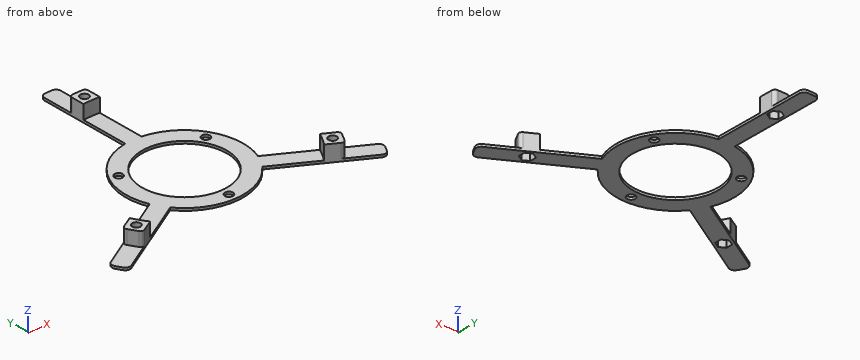
```python
from build123d import *

# Parameters (mm, degrees)
F0_R     = 2.5
F1_DEPTH = 1.5
F2_DEPTH = 10
F3_R     = 2
F4_R     = 3
F5_DEPTH = 4.5


with BuildPart() as f1:
    # F0 (on Top) → F1 (new body)
    with BuildSketch(Plane.XY):
        with BuildLine():
            Line((84.6583836258, -43.1040378836), (67.3074069841, -33.0864468488))
            ThreePointArc((67.3074069841, -33.0864468488), (64.9519052838, -37.5), (62.3074069841, -41.7467008867))
            Line((62.3074069841, -41.7467008867), (79.6583836258, -51.7642919214))
            ThreePointArc((79.6583836258, -51.7642919214), (82.2724133595, -47.5), (84.6583836258, -43.1040378836))
        make_face()
        with BuildLine():
            ThreePointArc((62.3074069841, -41.7467008867), (64.9519052838, -37.5), (67.3074069841, -33.0864468488))
            Line((67.3074069841, -33.0864468488), (62.3074069841, -41.7467008867))
        make_face()
        with BuildLine():
            Line((67.3074069841, -33.0864468488), (58.6248608016, -28.0735764731))
            ThreePointArc((58.6248608016, -28.0735764731), (56.291651246, -32.5), (53.6248608016, -36.733830511))
            Line((53.6248608016, -36.733830511), (62.3074069841, -41.7467008867))
            Line((62.3074069841, -41.7467008867), (67.3074069841, -33.0864468488))
        make_face()
        Polygon((63.9661338928, -36.9308646221), (60.4661338928, -38.9515905642), (56.9661338928, -36.9308646221), (56.9661338928, -32.8894127377), (60.4661338928, -30.8686867956), (63.9661338928, -32.8894127377), align=None, mode=Mode.SUBTRACT)
        with BuildLine():
            Line((58.6248608016, -28.0735764731), (33.3747469625, -13.4954164511))
            ThreePointArc((33.3747469625, -13.4954164511), (31.1769145362, -18), (28.3747469625, -22.1556704889))
            Line((28.3747469625, -22.1556704889), (53.6248608016, -36.733830511))
            ThreePointArc((53.6248608016, -36.733830511), (56.291651246, -32.5), (58.6248608016, -28.0735764731))
        make_face()
        with BuildLine():
            Line((33.3747469625, -13.4954164511), (24.596379794, -8.4272238033))
            ThreePointArc((24.596379794, -8.4272238033), (22.5166604984, -13), (19.596379794, -17.0874778411))
            Line((19.596379794, -17.0874778411), (28.3747469625, -22.1556704889))
            ThreePointArc((28.3747469625, -22.1556704889), (31.1769145362, -18), (33.3747469625, -13.4954164511))
        make_face()
        with BuildLine():
            ThreePointArc((5, 25.5147016443), (20.0748598999, 16.5227116419), (26, 0))
            ThreePointArc((26, 0), (25.6466944716, -4.2716580713), (24.596379794, -8.4272238033))
            Line((24.596379794, -8.4272238033), (33.3747469625, -13.4954164511))
            ThreePointArc((33.3747469625, -13.4954164511), (35.3375925231, -6.8741948383), (36, 0))
            ThreePointArc((36, 0), (27.1661554144, 23.622023622), (5, 35.65108694))
            Line((5, 35.65108694), (5, 25.5147016443))
        make_face()
        with Locations((26.8467875173, 15.5)):
            Circle(F0_R, mode=Mode.SUBTRACT)
        with BuildLine():
            Line((28.3747469625, -22.1556704889), (19.596379794, -17.0874778411))
            ThreePointArc((19.596379794, -17.0874778411), (0, -26), (-19.596379794, -17.0874778411))
            Line((-19.596379794, -17.0874778411), (-28.3747469625, -22.1556704889))
            ThreePointArc((-28.3747469625, -22.1556704889), (0, -36), (28.3747469625, -22.1556704889))
        make_face()
        with Locations((0, -31)):
            Circle(F0_R, mode=Mode.SUBTRACT)
        with BuildLine():
            ThreePointArc((-28.3747469625, -22.1556704889), (-31.1769145362, -18), (-33.3747469625, -13.4954164511))
            Line((-33.3747469625, -13.4954164511), (-58.6248608016, -28.0735764731))
            ThreePointArc((-58.6248608016, -28.0735764731), (-56.291651246, -32.5), (-53.6248608016, -36.733830511))
            Line((-53.6248608016, -36.733830511), (-28.3747469625, -22.1556704889))
        make_face()
        with BuildLine():
            ThreePointArc((-19.596379794, -17.0874778411), (-22.5166604984, -13), (-24.596379794, -8.4272238033))
            Line((-24.596379794, -8.4272238033), (-33.3747469625, -13.4954164511))
            ThreePointArc((-33.3747469625, -13.4954164511), (-31.1769145362, -18), (-28.3747469625, -22.1556704889))
            Line((-28.3747469625, -22.1556704889), (-19.596379794, -17.0874778411))
        make_face()
        with BuildLine():
            ThreePointArc((-53.6248608016, -36.733830511), (-56.291651246, -32.5), (-58.6248608016, -28.0735764731))
            Line((-58.6248608016, -28.0735764731), (-67.3074069841, -33.0864468488))
            Line((-67.3074069841, -33.0864468488), (-62.3074069841, -41.7467008867))
            Line((-62.3074069841, -41.7467008867), (-53.6248608016, -36.733830511))
        make_face()
        Polygon((-63.9661338928, -32.8894127377), (-60.4661338928, -30.8686867956), (-56.9661338928, -32.8894127377), (-56.9661338928, -36.9308646221), (-60.4661338928, -38.9515905642), (-63.9661338928, -36.9308646221), align=None, mode=Mode.SUBTRACT)
        with BuildLine():
            Line((-62.3074069841, -41.7467008867), (-67.3074069841, -33.0864468488))
            ThreePointArc((-67.3074069841, -33.0864468488), (-64.9519052838, -37.5), (-62.3074069841, -41.7467008867))
        make_face()
        with BuildLine():
            ThreePointArc((-62.3074069841, -41.7467008867), (-64.9519052838, -37.5), (-67.3074069841, -33.0864468488))
            Line((-67.3074069841, -33.0864468488), (-84.6583836258, -43.1040378836))
            ThreePointArc((-84.6583836258, -43.1040378836), (-82.2724133595, -47.5), (-79.6583836258, -51.7642919214))
            Line((-79.6583836258, -51.7642919214), (-62.3074069841, -41.7467008867))
        make_face()
        with BuildLine():
            ThreePointArc((-24.596379794, -8.4272238033), (-22.5166604984, 13), (-5, 25.5147016443))
            Line((-5, 25.5147016443), (-5, 35.65108694))
            ThreePointArc((-5, 35.65108694), (-31.1769145362, 18), (-33.3747469625, -13.4954164511))
            Line((-33.3747469625, -13.4954164511), (-24.596379794, -8.4272238033))
        make_face()
        with Locations((-26.8467875173, 15.5)):
            Circle(F0_R, mode=Mode.SUBTRACT)
        with BuildLine():
            ThreePointArc((-5, 25.5147016443), (0, 26), (5, 25.5147016443))
            Line((5, 25.5147016443), (5, 35.65108694))
            ThreePointArc((5, 35.65108694), (0, 36), (-5, 35.65108694))
            Line((-5, 35.65108694), (-5, 25.5147016443))
        make_face()
        with BuildLine():
            ThreePointArc((-5, 35.65108694), (0, 36), (5, 35.65108694))
            Line((5, 35.65108694), (5, 64.8074069841))
            ThreePointArc((5, 64.8074069841), (0, 65), (-5, 64.8074069841))
            Line((-5, 64.8074069841), (-5, 35.65108694))
        make_face()
        with BuildLine():
            ThreePointArc((-5, 64.8074069841), (0, 65), (5, 64.8074069841))
            Line((5, 64.8074069841), (5, 74.8331477355))
            Line((5, 74.8331477355), (-5, 74.8331477355))
            Line((-5, 74.8331477355), (-5, 64.8074069841))
        make_face()
        Polygon((0, 73.8617292441), (3.5, 71.8410033019), (3.5, 67.7995514176), (0, 65.7788254755), (-3.5, 67.7995514176), (-3.5, 71.8410033019), align=None, mode=Mode.SUBTRACT)
        with BuildLine():
            Line((-5, 74.8331477355), (5, 74.8331477355))
            ThreePointArc((5, 74.8331477355), (0, 75), (-5, 74.8331477355))
        make_face()
        with BuildLine():
            ThreePointArc((-5, 74.8331477355), (0, 75), (5, 74.8331477355))
            Line((5, 74.8331477355), (5, 94.8683298051))
            ThreePointArc((5, 94.8683298051), (0, 95), (-5, 94.8683298051))
            Line((-5, 94.8683298051), (-5, 74.8331477355))
        make_face()
        Polygon((56.9661338928, -36.9308646221), (60.4661338928, -38.9515905642), (63.9661338928, -36.9308646221), (63.9661338928, -32.8894127377), (60.4661338928, -30.8686867956), (56.9661338928, -32.8894127377), align=None)
        with Locations((60.4661338928, -34.9101386799)):
            Circle(F0_R, mode=Mode.SUBTRACT)
        Polygon((3.5, 67.7995514176), (3.5, 71.8410033019), (0, 73.8617292441), (-3.5, 71.8410033019), (-3.5, 67.7995514176), (0, 65.7788254755), align=None)
        with Locations((0, 69.8202773598)):
            Circle(F0_R, mode=Mode.SUBTRACT)
        Polygon((-56.9661338928, -32.8894127377), (-60.4661338928, -30.8686867956), (-63.9661338928, -32.8894127377), (-63.9661338928, -36.9308646221), (-60.4661338928, -38.9515905642), (-56.9661338928, -36.9308646221), align=None)
        with Locations((-60.4661338928, -34.9101386799)):
            Circle(F0_R, mode=Mode.SUBTRACT)
    extrude(amount=F1_DEPTH)

    # F0 (on Top) → F2 (join)
    with BuildSketch(Plane.XY):
        with BuildLine():
            ThreePointArc((-53.6248608016, -36.733830511), (-56.291651246, -32.5), (-58.6248608016, -28.0735764731))
            Line((-58.6248608016, -28.0735764731), (-67.3074069841, -33.0864468488))
            Line((-67.3074069841, -33.0864468488), (-62.3074069841, -41.7467008867))
            Line((-62.3074069841, -41.7467008867), (-53.6248608016, -36.733830511))
        make_face()
        Polygon((-63.9661338928, -32.8894127377), (-60.4661338928, -30.8686867956), (-56.9661338928, -32.8894127377), (-56.9661338928, -36.9308646221), (-60.4661338928, -38.9515905642), (-63.9661338928, -36.9308646221), align=None, mode=Mode.SUBTRACT)
        with BuildLine():
            ThreePointArc((-5, 64.8074069841), (0, 65), (5, 64.8074069841))
            Line((5, 64.8074069841), (5, 74.8331477355))
            Line((5, 74.8331477355), (-5, 74.8331477355))
            Line((-5, 74.8331477355), (-5, 64.8074069841))
        make_face()
        Polygon((0, 73.8617292441), (3.5, 71.8410033019), (3.5, 67.7995514176), (0, 65.7788254755), (-3.5, 67.7995514176), (-3.5, 71.8410033019), align=None, mode=Mode.SUBTRACT)
        with BuildLine():
            Line((67.3074069841, -33.0864468488), (58.6248608016, -28.0735764731))
            ThreePointArc((58.6248608016, -28.0735764731), (56.291651246, -32.5), (53.6248608016, -36.733830511))
            Line((53.6248608016, -36.733830511), (62.3074069841, -41.7467008867))
            Line((62.3074069841, -41.7467008867), (67.3074069841, -33.0864468488))
        make_face()
        Polygon((63.9661338928, -36.9308646221), (60.4661338928, -38.9515905642), (56.9661338928, -36.9308646221), (56.9661338928, -32.8894127377), (60.4661338928, -30.8686867956), (63.9661338928, -32.8894127377), align=None, mode=Mode.SUBTRACT)
        Polygon((-56.9661338928, -32.8894127377), (-60.4661338928, -30.8686867956), (-63.9661338928, -32.8894127377), (-63.9661338928, -36.9308646221), (-60.4661338928, -38.9515905642), (-56.9661338928, -36.9308646221), align=None)
        with Locations((-60.4661338928, -34.9101386799)):
            Circle(F0_R, mode=Mode.SUBTRACT)
        Polygon((56.9661338928, -36.9308646221), (60.4661338928, -38.9515905642), (63.9661338928, -36.9308646221), (63.9661338928, -32.8894127377), (60.4661338928, -30.8686867956), (56.9661338928, -32.8894127377), align=None)
        with Locations((60.4661338928, -34.9101386799)):
            Circle(F0_R, mode=Mode.SUBTRACT)
        Polygon((3.5, 67.7995514176), (3.5, 71.8410033019), (0, 73.8617292441), (-3.5, 71.8410033019), (-3.5, 67.7995514176), (0, 65.7788254755), align=None)
        with Locations((0, 69.8202773598)):
            Circle(F0_R, mode=Mode.SUBTRACT)
    extrude(amount=F2_DEPTH)

    # F3
    f3_edges = [f1.edges().sort_by_distance(p)[0] for p in [
        (67.307407, -33.086447, 5.75),
        (62.307407, -41.746701, 5.75),
        (-62.307407, -41.746701, 5.75),
        (-67.307407, -33.086447, 5.75),
        (5, 74.833148, 5.75),
        (-5, 74.833148, 5.75),
    ]]
    fillet(f3_edges, radius=F3_R)

    # F4
    f4_edges = [f1.edges().sort_by_distance(p)[0] for p in [
        (84.658384, -43.104038, 0.75),
        (79.658384, -51.764292, 0.75),
        (-79.658384, -51.764292, 0.75),
        (-84.658384, -43.104038, 0.75),
        (-5, 94.86833, 0.75),
        (5, 94.86833, 0.75),
    ]]
    fillet(f4_edges, radius=F4_R)

    # F0 (on Top) → F5 (cut)
    with BuildSketch(Plane.XY):
        Polygon((56.9661338928, -36.9308646221), (60.4661338928, -38.9515905642), (63.9661338928, -36.9308646221), (63.9661338928, -32.8894127377), (60.4661338928, -30.8686867956), (56.9661338928, -32.8894127377), align=None)
        with Locations((60.4661338928, -34.9101386799)):
            Circle(F0_R, mode=Mode.SUBTRACT)
        Polygon((-56.9661338928, -32.8894127377), (-60.4661338928, -30.8686867956), (-63.9661338928, -32.8894127377), (-63.9661338928, -36.9308646221), (-60.4661338928, -38.9515905642), (-56.9661338928, -36.9308646221), align=None)
        with Locations((-60.4661338928, -34.9101386799)):
            Circle(F0_R, mode=Mode.SUBTRACT)
        Polygon((3.5, 67.7995514176), (3.5, 71.8410033019), (0, 73.8617292441), (-3.5, 71.8410033019), (-3.5, 67.7995514176), (0, 65.7788254755), align=None)
        with Locations((0, 69.8202773598)):
            Circle(F0_R, mode=Mode.SUBTRACT)
    extrude(amount=F5_DEPTH, mode=Mode.SUBTRACT)


solid = f1.part
```
Geometry: final body of the model. Coordinates: model frame, mm. Round coordinates to 2 decimals unless told otherwise and drop trailing zeros. Write each loop counter-clockwise with the first axis right and the second up, starting at its lowest first coordinate (ties: lowest second). Pieces come first, ordered by that corner, then holes. Notation, with made-up numbers: (39, 35.25) -> (76, 35.25) arc R23 ccw to (76, 50.25) -> close; hole circle Ø3 at (71.25, 61). An arc over 180 degrees is marked (long way). Return JSON: item names as keys, results as strings.
Q1. Ray query, line 1 (Y direction, x = 0, z = 0.9); line 2 (X direction, y = -31, z = 2.5); line 3 (Z direction, x = 4, y = 52.5). Return the intervals inside material, ascending.
From the geometry:
{"line 1": "-36 to -33.5, -28.5 to -26, 26 to 65.78, 73.86 to 95", "line 2": "-63.69 to -60.69, -60.24 to -57.13, 57.13 to 60.24, 60.69 to 63.69", "line 3": "0 to 1.5"}
Q2. First-contact query: pin 1 Ø3 at (x, z) = (52, 1.5) entering from -Y; pin 2 Ø5 at (x, z) = (0.5, 7) entering from +Y; pin 3 Ø20.5 at (x, y) = (69.5, -43.5) entering from +Z; pin 4 Ø4 at (x, y) = (26.85, 15.5) entering from -Z. Flat tips, straight axial feed; report the tip coordinate or a pass-through.
From the geometry:
{"pin 1": "y = -36.66", "pin 2": "y = 74.83", "pin 3": "z = 10", "pin 4": "through"}
Q3. Section A-A on z = 6.5. Return the cut outline in (x, y).
From the geometry:
{"outline": "(-66.31, -34.82) -> (-63.31, -40.01) arc R2 ccw to (-60.58, -40.75) -> (-53.62, -36.73) arc R65 cw to (-58.62, -28.07) -> (-65.58, -32.09) arc R2 ccw to start; (-5, 64.81) arc R65 cw to (5, 64.81) -> (5, 72.83) arc R2 ccw to (3, 74.83) -> (-3, 74.83) arc R2 ccw to (-5, 72.83) -> close; (53.62, -36.73) -> (60.58, -40.75) arc R2 ccw to (63.31, -40.01) -> (66.31, -34.82) arc R2 ccw to (65.58, -32.09) -> (58.62, -28.07) arc R65 cw to start; hole circle Ø5 at (-60.47, -34.91); hole circle Ø5 at (0, 69.82); hole circle Ø5 at (60.47, -34.91)"}
Q4. Section C-C on y = 15.5. Return the cut outline in (x, z), and give its area (3 significant figures).
From the geometry:
{"outline": "(-32.49, 0) -> (-29.35, 0) -> (-29.35, 1.5) -> (-32.49, 1.5) -> close; (-24.35, 0) -> (-20.87, 0) -> (-20.87, 1.5) -> (-24.35, 1.5) -> close; (20.87, 0) -> (24.35, 0) -> (24.35, 1.5) -> (20.87, 1.5) -> close; (29.35, 0) -> (32.49, 0) -> (32.49, 1.5) -> (29.35, 1.5) -> close", "area": "19.9 mm2"}
Q5. Section B-B on x = 9. Return the cut outline in (y, z), and give its area (3 significant figures).
From the geometry:
{"outline": "(-34.86, 0) -> (-24.39, 0) -> (-24.39, 1.5) -> (-34.86, 1.5) -> close; (24.39, 0) -> (34.86, 0) -> (34.86, 1.5) -> (24.39, 1.5) -> close", "area": "31.4 mm2"}
Q6. Section D-D on y = 50. Return the cut outline in (x, z).
From the geometry:
{"outline": "(-5, 0) -> (5, 0) -> (5, 1.5) -> (-5, 1.5) -> close"}
